Read the model definition and answer for the solid it produces. Units are mm, in the model's axes. A direction names the side the tool comes from. Coordinates: 2 decimals unless noted, no trailing zeros. Write each loop counter-clockwise with the first axis right and the second up, starting at its lowest first coordinate (ties: lowest second). Pieces come first, ordered by that corner, then holes.
1) Determine the mould class of faces 4 (the face through (35.69, 0.83, 11)), 5 (the face through (0, 0, 0)), 6 (the face through (12.28, -1.306, 4.056)) for opening direction X: +X half, -X half, draft (parallel to the pull), parting line (faces both ways), or undercut.
2) The part is cut by section B-B (z = 4.75). Give the number of separate pieces and of enclosed holes in the cut face, then the cut area to 3 significant figures.
3) Find the intervals of material crossed by line 1 (X direction, y = -0.5, z = 1); line 2 (X direction, y = 2.25, z = 5.75); line 3 (X direction, y = 0.25, z = 10.5), in increasing order.
4) Each of these flat-tipped pins is pushed along its axis until it touches: pin 1 Ø1 at (y, z) = (0, 3) entering from +X; pin 2 Ø4 at (y, z) = (-2, 6.5) entering from +X. Where does it stop, or does it pass through?
5) The part is cut by section A-A (x = 6). Determine the outline of the cut face in (y, z).
6) Which of the six approach directions +Z, -Z, +X, -X, +Y, -Y give full straight-line access (tool end or side, diameter ignored) to faces 1 (the face through (-10.5, 0.1, 6)), 2 (the face through (-15, -2.575, 4)), 3 (the face through (24.287, -0.07, 5.53))?
from build123d import *

# Parameters (mm, degrees)
F1_DEPTH  = 4
F2_R      = 3.99999
F4_DEPTH  = 8
F6_DEPTH  = 4
F9_R      = 4
F10_DEPTH = 6.851053331
F12_SIZE2 = 1
F12_SIZE  = 3.7320508076


# Not quite as in the source:
# - a fillet or chamfer is up to 0.001 mm smaller than in the source, because OpenCascade refuses the exact size


with BuildPart() as f1:
    # F0 (on Front) → F1 (new body, symmetric)
    with BuildSketch(Plane.XZ):
        Polygon((-26.6568542495, 0), (0, 0), (0, 8), (-34.6568542495, 8), align=None)
    extrude(amount=F1_DEPTH, both=True)

    # F2 (radius 4 in the source; OpenCascade refuses exactly that, so slightly less here)
    f2_edges = [f1.edges().sort_by_distance(p)[0] for p in [
        (-30.656854, 4, 4),
        (-30.656854, -4, 4),
    ]]
    fillet(f2_edges, radius=F2_R)

    # F3 (on face) → F4 (cut, through all)
    with BuildSketch(Plane.XY.offset(8)):
        Polygon((-11.5266461137, 0), (-13.0133230568, 2.575), (-15.9866769432, 2.575), (-17.4733538863, 0), (-15.9866769432, -2.575), (-13.0133230568, -2.575), align=None)
    extrude(amount=-F4_DEPTH, mode=Mode.SUBTRACT)

    # F5 (on face) → F6 (cut)
    with BuildSketch(Plane.XY.offset(8)):
        with BuildLine():
            ThreePointArc((-14.5, 4), (-10.5, 0), (-14.5, -4))
            Line((-14.5, -4), (0, -4))
            Line((0, -4), (0, 4))
            Line((0, 4), (-14.5, 4))
        make_face()
    extrude(amount=-F6_DEPTH, mode=Mode.SUBTRACT)

    # F9 (on line) → F10 (join, symmetric)
    with BuildSketch(Plane(origin=(-18.5, 0, 18.5), x_dir=(0, 1, 0), z_dir=(0.7071067812, 0, -0.7071067812))):
        with Locations((0, -14.8492424049)):
            Circle(F9_R)
    extrude(amount=F10_DEPTH, both=True)

    # F7 (on Front) → F11 (revolve, cut)
    with BuildSketch(Plane.XZ):
        Polygon((-11.4302859145, -11.8147781158), (-10.3077538993, -10.6922461007), (-44.6173825807, 23.6173825807), (-45.7399145958, 22.4948505656), align=None)
    revolve(axis=Axis((-27.46256824, 0, 6.46256824), (-0.7071067812, 0, 0.7071067812)), mode=Mode.SUBTRACT)

    # F12
    f12_edges = [f1.edges().sort_by_distance(p)[0] for p in [
        (-32.721894, 0, 13.966958),
    ]]
    f12_side = f1.faces().sort_by_distance((-25.685621, 0, 6.930685))[0]
    chamfer(f12_edges, length=F12_SIZE, length2=F12_SIZE2, reference=f12_side)

    # F13: F1 across face


with BuildPart() as f1_1:
    add(f1.part)
    add(f1.part.mirror(Plane(origin=(0, 0, 2), x_dir=(0, 1, 0), z_dir=(1, 0, 0))))


solid = f1_1.part
Reported:
1. face 4: +X half
1. face 5: draft
1. face 6: undercut
2. separate pieces: 2
2. enclosed holes: 4
2. area: 233 mm2
3. line 1: x = -27.61 to -24.13, -19.87 to -17.18, -11.82 to 11.82, 17.18 to 19.87, 24.13 to 27.61
3. line 2: x = -31.43 to -16.17, -12.83 to -11.19, 11.19 to 12.83, 16.17 to 31.43
3. line 3: x = -36.19 to -34.76, -29.28 to -25.85, 25.85 to 29.28, 34.76 to 36.19
4. pin 1: stops at x = 30.16
4. pin 2: stops at x = 34.73
5. outline: (-4, 0) - (4, 0) - (4, 4) - (-4, 4) - close
6. face 1: +Z
6. face 2: +Z, -Z
6. face 3: none
